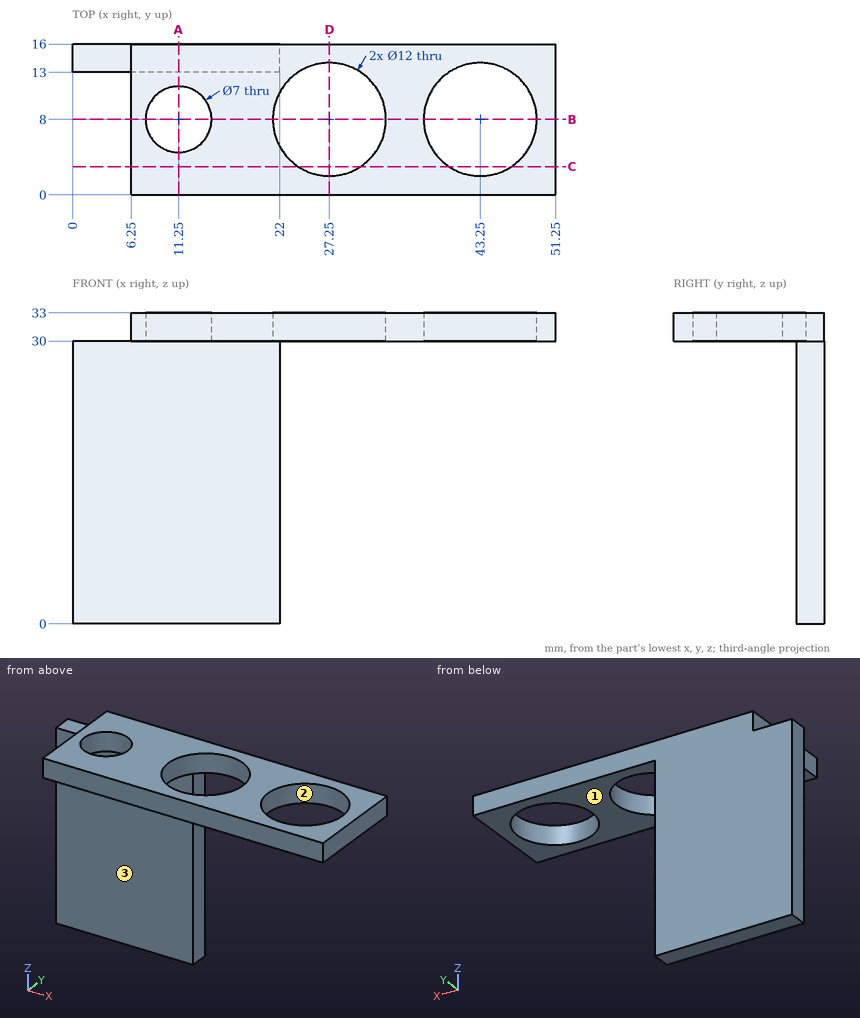
Source: three-view drawing plus pictorial views. Frame: mm from the lowest corner of the part. Coordinates: 2 decimals unless noted, no trailing zeros. Loops run counter-clockwise (first coordinate to the right, second up) from the corner with the lowest first, then second, coordinate; pieces in that order, holes last. Notation, with made-up numbers: (-0.75, 43) -> (49.25, 43) arc R23 ccw to (49.25, 57) -> close; hole circle Ø7 at (33, 87). An arc over 180 degrees is marked (long way). Write each question's results on one line, items separated by ' | '. Start each with the question number.
Q1. Section C-C, the plane y = 3. Return the cut outline in (x, z), plus the area to 3 significant figures.
Q2. Ray query, line 1 (X direction, y = 9.25, z = 31.5); line 2 (Y direction, x = 27.25, z = 30.9); line 3 (Y direction, x = 11.25, z = 31.9). Return the intervals inside material, ascending. Write a range as from..to.
Q3. Section D-D, the plane x = 27.25. Return the cut outline in (y, z).
Q4. Section A-A, the plane x = 11.25. Return the cut outline in (y, z), plus the area to 3 significant figures.
Q5. Section B-B, the plane y = 8. Return the cut outline in (x, z).
Q6. Pin query (flat end, axial travel): pin 1 (5 mm diameter, centred on x = 37, y = 13, fed in from -Z); pin 2 (0.9 mm diameter, centred on x = 3.5, y = 14, fed in from +Z); pin 3 (12 mm diameter, centred on x = 8.5, z = 7.5, fed in from -Y). Return the tip coordinate at first contact, or that it passes through.
Q7. Pull-direction query (Y, two-part tool) for the marked faces 1, 2 and 3; classes: released by +Y, released by -Y, zero draft, split by the parting line, or undercut.
Found:
1) outline: (6.25, 30) -> (23.93, 30) -> (23.93, 33) -> (6.25, 33) -> close; (30.57, 30) -> (39.93, 30) -> (39.93, 33) -> (30.57, 33) -> close; (46.57, 30) -> (51.25, 30) -> (51.25, 33) -> (46.57, 33) -> close | area: 95.2 mm2
2) line 1: 6.25..7.98, 14.52..21.38, 33.12..37.38, 49.12..51.25 | line 2: 0..2, 14..16 | line 3: 0..4.5, 11.5..16
3) outline: (0, 30) -> (2, 30) -> (2, 33) -> (0, 33) -> close; (14, 30) -> (16, 30) -> (16, 33) -> (14, 33) -> close
4) outline: (0, 30) -> (4.5, 30) -> (4.5, 33) -> (0, 33) -> close; (11.5, 30) -> (13, 30) -> (13, 0) -> (16, 0) -> (16, 33) -> (11.5, 33) -> close | area: 117 mm2
5) outline: (6.25, 30) -> (7.75, 30) -> (7.75, 33) -> (6.25, 33) -> close; (14.75, 30) -> (21.25, 30) -> (21.25, 33) -> (14.75, 33) -> close; (33.25, 30) -> (37.25, 30) -> (37.25, 33) -> (33.25, 33) -> close; (49.25, 30) -> (51.25, 30) -> (51.25, 33) -> (49.25, 33) -> close
6) pin 1: z = 30 | pin 2: z = 30 | pin 3: y = 13
7) face 1: zero draft | face 2: undercut | face 3: released by -Y
